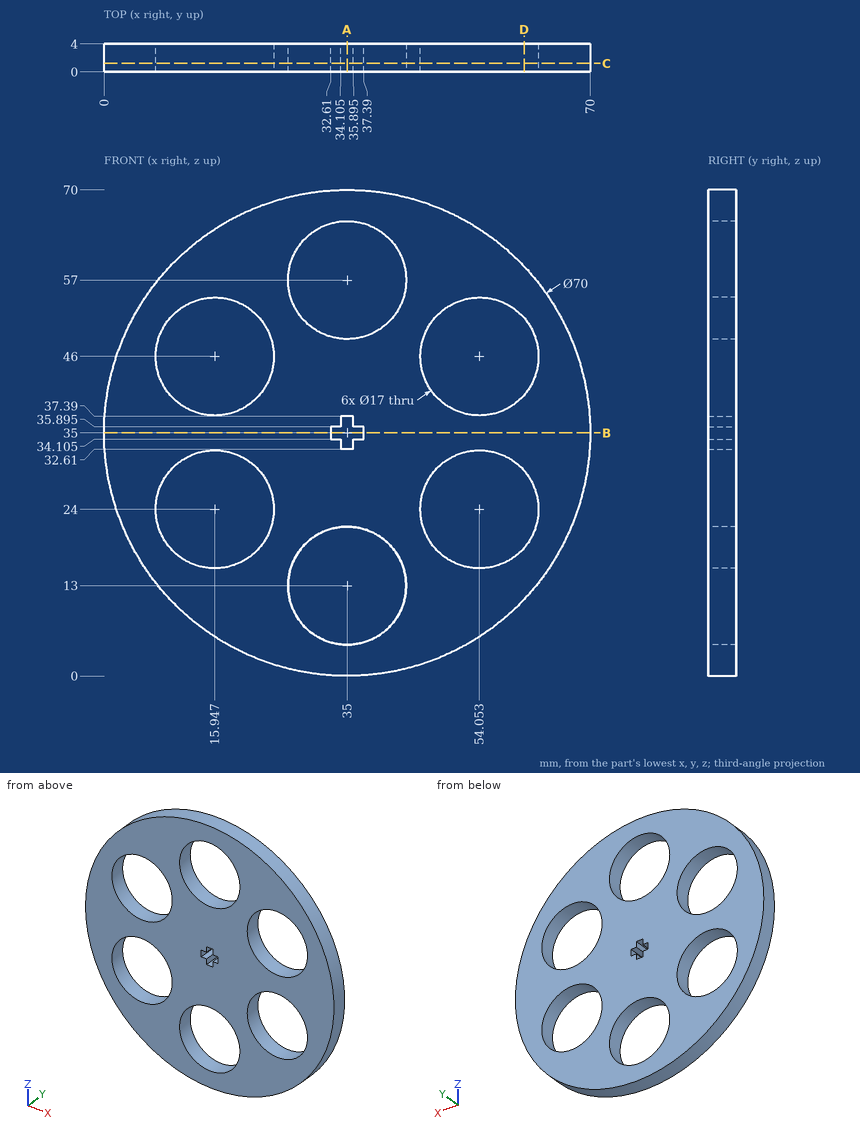
Geometry: see drawing. Coordinates: mm, zero at the bounding-box minimum. Coordinates: 2 decimals unless noted, no trailing zeros. Loops run counter-clockwise (first coordinate to the right, second up) from the corner with the lowest first, then second, coordinate; pieces in that order, holes last. Notation, with made-up numbers: (-5, 33.5) - (29, 33.5) arc R28 ccw to (29, 61.5) - close; hole circle Ø2 at (49, 41). An arc over 180 degrees is marked (long way). Put each result on its own line as item: value. Start each with the question number.
Q1. Pin query (flat end, axial travel): pin 1 Ø1.5 at (x, y) = (32, 1.5) entering from +Z; pin 2 Ø0.5 at (y, z) = (2, 35.5) entering from -X; pin 3 Ø0.7 at (x, y) = (36.5, 2.5) entering from +Z. Return the tip coordinate at first contact, or that it passes through.
Q2. Cut plane C-C, the plane y = 1.2. Return loops of the section in (x, z) (1 decimal), and give its area (3 significant figures).
Q3. Line query: line 1 (Z direction, x = 35, y = 2.2); line 2 (Z direction, x = 29, y = 2.9); line 3 (Z direction, x = 30.5, y = 2.4). Output: solid intervals per line, ascending.
Q4. Cut plane A-A, the plane x = 35. Return loops of the section in (y, z).
Q5. Cut plane B-B, the plane z = 35. Return loops of the section in (x, y), and give its area (3 significant figures).
Q6. Cut plane D-D, the plane x = 60.5. Return loops of the section in (y, z).
Filled sheet:
1. pin 1: z = 69.93
1. pin 2: x = 0
1. pin 3: z = 69.98
2. outline: circle Ø70 at (35, 35); hole circle Ø17 at (15.9, 24); hole circle Ø17 at (15.9, 46); hole circle Ø17 at (35, 13); hole circle Ø17 at (35, 57); hole (32.6, 34.1) - (34.1, 34.1) - (34.1, 32.6) - (35.9, 32.6) - (35.9, 34.1) - (37.4, 34.1) - (37.4, 35.9) - (35.9, 35.9) - (35.9, 37.4) - (34.1, 37.4) - (34.1, 35.9) - (32.6, 35.9) - close; hole circle Ø17 at (54.1, 24); hole circle Ø17 at (54.1, 46)
2. area: 2,470 mm²
3. line 1: 0 to 4.5, 21.5 to 32.61, 37.39 to 48.5, 65.5 to 70
3. line 2: 0.52 to 6.98, 19.02 to 50.98, 63.02 to 69.48
3. line 3: 0.29 to 5.79, 20.21 to 49.79, 64.21 to 69.71
4. outline: (0, 0) - (4, 0) - (4, 4.5) - (0, 4.5) - close; (0, 21.5) - (4, 21.5) - (4, 32.61) - (0, 32.61) - close; (0, 37.39) - (4, 37.39) - (4, 48.5) - (0, 48.5) - close; (0, 65.5) - (4, 65.5) - (4, 70) - (0, 70) - close
5. outline: (0, 0) - (32.61, 0) - (32.61, 4) - (0, 4) - close; (37.39, 0) - (70, 0) - (70, 4) - (37.39, 4) - close
5. area: 261 mm²
6. outline: (0, 11.03) - (4, 11.03) - (4, 18.46) - (0, 18.46) - close; (0, 29.54) - (4, 29.54) - (4, 40.46) - (0, 40.46) - close; (0, 51.54) - (4, 51.54) - (4, 58.97) - (0, 58.97) - close
